Study the drawing (mm; zero at the part's minimum x, y, z) and answer. A direction names the side the tool comes from. Round coordinates to 2 decimals unless told otherwise and drop trailing zeros. Order: outer loops, then holes, each group sorted by start corner. A loop starts at its lowest first (then second) coordinate and runs counter-clockwise, first axis right, second up. Notation, with made-up numbers: (-30, -25) - (17, -25) arc R22 ccw to (17, -15) - close; hole circle Ø10 at (39, -9.75). An arc over 180 degrees is marked (long way). Put each result on its own line as item: value. Start each with the question number.
Q1. Section C-C on y = 11 is taken. Give the vertices of the cut face in (x, z).
Q2. Which of the six approach directions +Z, -Z, +X, -X, +Y, -Y give full straight-line access (tool end or side, diameter ignored) to the marked faces 1 and 2?
Q3. Section A-A on x = 13.4 is taken. Give the vertices of the cut face in (y, z), then the cut area to 3 significant figures.
Q4. Find the intervals of material crossed by line 1 along X through (y, z) = (1, 36); line 2 along X through (y, z) = (4, 7.5); line 3 along Y through (x, z) = (25.45, 6), in increasing order. Write a range as from..to.
Q5. Section B-B on z = 8 is taken. Give the vertices of the cut face in (x, y).
Q6. For a pull along X with two mould halves and no side action, classify the marked faces 3, 4 and 5 as pulls with the +X half, pulls with the -X half, needs draft (parallel to the pull), parting line crosses it, or undercut.
Q7. Each of these flat-tipped pins is pushed along its axis until it touches: pin 1 Ø5 at (x, z) = (21.4, 36) entering from -Y; pin 2 Ø1.8 at (x, z) = (13.4, 8) entering from +Y. Where does it stop, or does it pass through?
Q8. Section D-D on x = 9.75 is taken. Give the vertices of the cut face in (y, z), then the cut area to 3 significant figures.
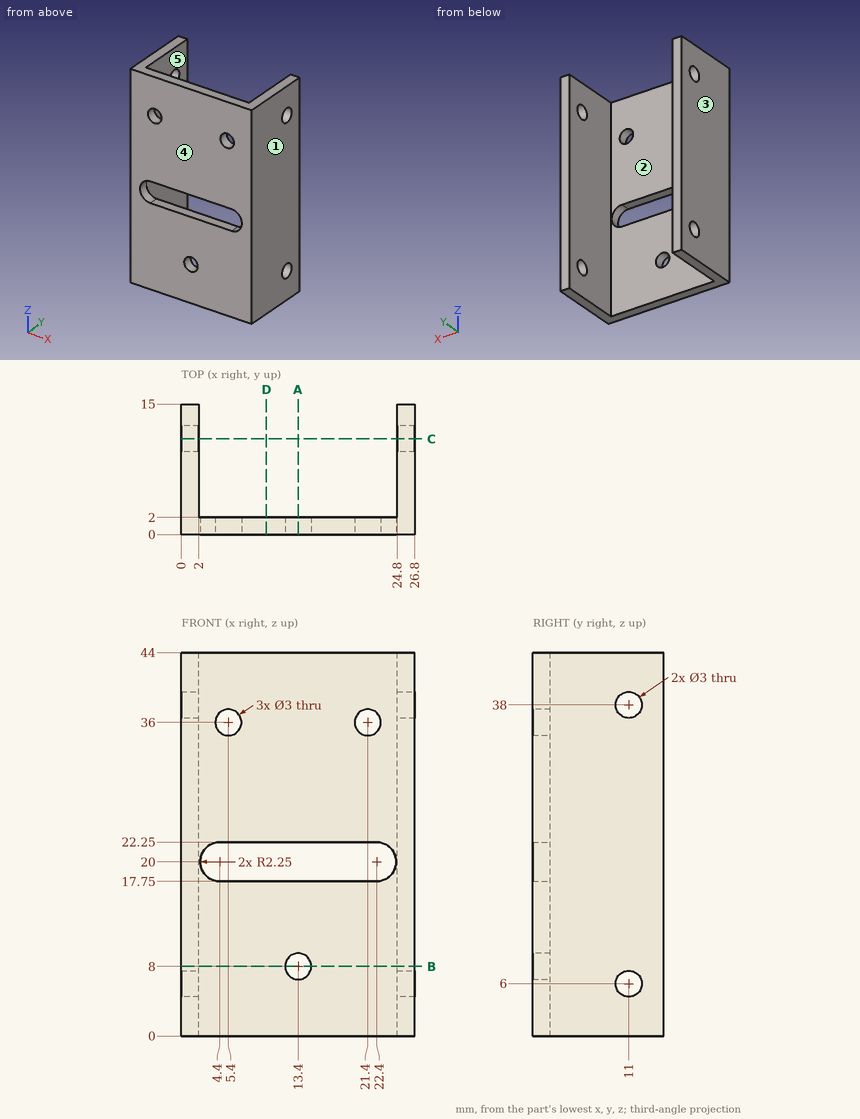
Findings:
1. outline: (0, 0) - (2, 0) - (2, 4.5) - (0, 4.5) - close; (0, 7.5) - (2, 7.5) - (2, 36.5) - (0, 36.5) - close; (0, 39.5) - (2, 39.5) - (2, 44) - (0, 44) - close; (24.8, 0) - (26.8, 0) - (26.8, 4.5) - (24.8, 4.5) - close; (24.8, 7.5) - (26.8, 7.5) - (26.8, 36.5) - (24.8, 36.5) - close; (24.8, 39.5) - (26.8, 39.5) - (26.8, 44) - (24.8, 44) - close
2. face 1: +Z, -Z, +X, +Y, -Y
2. face 2: +Z, -Z, +Y
3. outline: (0, 0) - (2, 0) - (2, 6.5) - (0, 6.5) - close; (0, 9.5) - (2, 9.5) - (2, 17.75) - (0, 17.75) - close; (0, 22.25) - (2, 22.25) - (2, 44) - (0, 44) - close
3. area: 73.0 mm2
4. line 1: 0..3.9, 6.9..19.9, 22.9..26.8
4. line 2: 0..2, 24.8..26.8
4. line 3: 0..9.5, 12.5..15
5. outline: (0, 0) - (11.9, 0) - (11.9, 2) - (2, 2) - (2, 15) - (0, 15) - close; (14.9, 0) - (26.8, 0) - (26.8, 15) - (24.8, 15) - (24.8, 2) - (14.9, 2) - close
6. face 3: pulls with the -X half
6. face 4: needs draft
6. face 5: undercut
7. pin 1: y = 0
7. pin 2: through
8. outline: (0, 0) - (2, 0) - (2, 17.75) - (0, 17.75) - close; (0, 22.25) - (2, 22.25) - (2, 44) - (0, 44) - close
8. area: 79.0 mm2
